from build123d import *

# Parameters (mm, degrees)
SKETCH_1_R          = 2.05
SKETCH_1_R_2        = 7.02
SKETCH_1_W          = 2.1
SKETCH_1_H          = 8.1
EXTRUDE_1_DEPTH     = 2
FILLET_1_R          = 2
SKETCH_3_R          = 2.05
SKETCH_3_R_2        = 2
CUT_EXTRUDE_1_DEPTH = 2


with BuildPart() as part:
    # 草图1 → 凸台-拉伸1 (new body)
    with BuildSketch(Plane.XY):
        with BuildLine():
            Line((230.542857143, -30.045714286), (199.556073527, -36.55591431))
            Line((199.556073527, -36.55591431), (192.746868021, -38.145714286))
            Line((192.746868021, -38.145714286), (21.365844759, -38.145714286))
            Line((21.365844759, -38.145714286), (2.692857143, -38.295714286))
            Line((2.692857143, -38.295714286), (2.692857143, -35.802553436))
            Line((2.692857143, -35.802553436), (-5.457142857, -35.802553436))
            Line((-5.457142857, -35.802553436), (-5.457142857, 41.704285714))
            Line((-5.457142857, 41.704285714), (7.542857143, 41.704285714))
            Line((7.542857143, 41.704285714), (7.542857143, 14.854285714))
            Line((7.542857143, 14.854285714), (16.542857143, 14.854285714))
            Line((16.542857143, 14.854285714), (16.542857143, 41.704285714))
            Line((16.542857143, 41.704285714), (199.542857143, 41.704285714))
            Line((199.542857143, 41.704285714), (230.542857143, 29.754285714))
            ThreePointArc((230.542857143, 29.754285714), (260.442857143, -0.145714286), (230.542857143, -30.045714286))
        make_face()
        with Locations((0.542857143, 29.854285714)):
            Circle(SKETCH_1_R, mode=Mode.SUBTRACT)
        with Locations((0.542857143, -0.145714286)):
            Circle(SKETCH_1_R, mode=Mode.SUBTRACT)
        with Locations((0.542857143, -30.145714286)):
            Circle(SKETCH_1_R, mode=Mode.SUBTRACT)
        with Locations((230.542857143, -0.145714286)):
            Circle(SKETCH_1_R_2, mode=Mode.SUBTRACT)
        with Locations((0.542857143, 14.854285714)):
            Rectangle(SKETCH_1_W, SKETCH_1_H, mode=Mode.SUBTRACT)
        with BuildLine():
            Line((59.099206329, 22.4106349), (50.542857143, 30.966984086))
            Line((50.542857143, 30.966984086), (19.430158771, -0.145714286))
            Line((19.430158771, -0.145714286), (50.542857143, -31.258412658))
            Line((50.542857143, -31.258412658), (81.655555515, -0.145714286))
            Line((81.655555515, -0.145714286), (73.099206329, 8.4106349))
            ThreePointArc((73.099206329, 8.4106349), (74.584487703, 23.895916275), (59.099206329, 22.4106349))
        make_face(mode=Mode.SUBTRACT)
        with Locations((0.542857143, -15.145714286)):
            Rectangle(SKETCH_1_W, SKETCH_1_H, mode=Mode.SUBTRACT)
    extrude(amount=EXTRUDE_1_DEPTH)

    # 圆角1
    fillet_1_edges = [part.edges().sort_by_distance(p)[0] for p in [
        (7.542857143, 41.704285714, 1),
        (7.542857143, 14.854285714, 1),
        (16.542857143, 14.854285714, 1),
        (16.542857143, 41.704285714, 1),
    ]]
    fillet(fillet_1_edges, radius=FILLET_1_R)

    # 草图3 → 切除-拉伸1 (cut)
    with BuildSketch(Plane.XY.offset(2)):
        with Locations((25.542857143, 35.704285714)):
            Circle(SKETCH_3_R)
        with Locations((110.542857143, 35.704285714)):
            Circle(SKETCH_3_R)
        with Locations((195.542857143, 35.704285714)):
            Circle(SKETCH_3_R)
        with Locations((110.542857143, -34.295714286)):
            Circle(SKETCH_3_R)
        with Locations((195.542857143, -34.295714286)):
            Circle(SKETCH_3_R)
        with Locations((25.542857143, -34.295714286)):
            Circle(SKETCH_3_R)
        with Locations((190.542857143, -0.145714286)):
            Circle(SKETCH_3_R_2)
        with Locations((140.542857143, 16.354285714)):
            Circle(SKETCH_3_R_2)
        with Locations(Location((140.542857143, -16.645714286, 0), (0, 0, 180))):
            Circle(SKETCH_3_R_2)
        Polygon((148.153334198, 25.704285714), (148.153334198, 9.632158315), (167.669488896, 25.704285714), align=None)
        Polygon((185.542857143, -24.295714286), (138.41622539, -24.295714286), (185.542857143, 14.51445304), align=None)
        Polygon((120.542857143, -13.105881612), (120.542857143, 25.704285714), (134.014872528, 25.704285714), (134.014872528, -2.011280706), align=None)
    extrude(amount=-CUT_EXTRUDE_1_DEPTH, mode=Mode.SUBTRACT)


solid = part.part
Part model, mm, in its own coordinate system. A direction names the side the tool comes from. Coordinates: 2 decimals unless noted, no trailing zeros. Order: outer loops, then holes, each group sorted by start corner. A loop starts at its lowest first (then second) coordinate and runs counter-clockwise, first axis right, second up. Notation, with made-up numbers: (33.25, -33.5) - (72.25, -33.5) arc R7 cw to (72.25, -21.5) - close; hole circle Ø10 at (47.5, 21.5). An arc over 180 degrees is marked (long way). Use CSV: the item, a comma, the result in double quotes.
Item 1: 3-axis set-ups, long thin cutter, end or side, ignore diameter. For faces 1 (the face through (260.436, 0.512, 0.986)), 2 (the face through (157.775, 17.556, 1.014)): which of +Z, -Z, +X, -X, +Y, -Y reach the whole face in a straight line?
Solved:
face 1,"+Z, -Z, +X"
face 2,"+Z, -Z"
Item 2: Mould opens along X. For faces 3 (the face through (237.24, 1.96, 0.99)), 4 (the face through (214.83, 35.81, 0.99)), 5 (the face through (129, -7, 2)) say: +X half, -X half, draft (parallel to the pull), parting line (faces both ways), or undercut.
Solved:
face 3,"undercut"
face 4,"+X half"
face 5,"draft"
Item 3: Drop flat-ended pins along their axis: P1, Ø3.5, axis at x = 0.54, y = -0.15, coming from the -Z side; P2, Ø0.6, axis at y = 19, z = 1, coming from the +X side. Give the stop position or say it passes through.
Solved:
P1,"passes through"
P2,"stops at x = 253.76"
Item 4: Probe probe 1 along Y at (x, z) = (140, 1.7); probe 2 along Y at (x, z) = (9.5, 1.3); probe 3 along X at (y, z) = (-3, 0.9). List the from-to ranges inside material, lowest first.
Solved:
probe 1,"y = -38.15 to -24.3, -22.99 to -18.57, -14.72 to 14.43, 18.28 to 41.7"
probe 2,"y = -38.24 to 14.85"
probe 3,"x = -5.46 to 22.28, 78.8 to 120.54, 132.81 to 164.28, 185.54 to 224.13, 236.96 to 260.31"
Item 5: Saw through at D-D on x = 182. Give the cut face in (y, z), and give its area (3 significant figures).
Solved:
outline,"(-38.15, 0) - (-24.3, 0) - (-24.3, 2) - (-38.15, 2) - close; (11.6, 0) - (41.7, 0) - (41.7, 2) - (11.6, 2) - close"
area,"87.9 mm²"
Item 6: Saw through at A-A on x = 30. Give the cut face in (y, z), and give its area (3 significant figures).
Solved:
outline,"(-38.15, 0) - (-10.72, 0) - (-10.72, 2) - (-38.15, 2) - close; (10.42, 0) - (41.7, 0) - (41.7, 2) - (10.42, 2) - close"
area,"117 mm²"
Item 7: Saw through at B-B on x = 151. Give the cut face in (y, z).
Solved:
outline,"(-38.15, 0) - (-24.3, 0) - (-24.3, 2) - (-38.15, 2) - close; (-13.93, 0) - (11.98, 0) - (11.98, 2) - (-13.93, 2) - close; (25.7, 0) - (41.7, 0) - (41.7, 2) - (25.7, 2) - close"
Item 8: Saw through at C-C on z = 0.65. Give the number of separate pieces and of enclosed holes in the cut face, and give its area (3 significant figures).
Solved:
separate pieces,"1"
enclosed holes,"19"
area,"15,600 mm²"
